Design review of the part shown in the three views and the two pictorial views. Dimensions are in mm from the part's minimum x, y and z. A direction names the side the tool comes from. Round coordinates to 2 decimals unless told otherwise and drop trailing zeros. Order: outer loops, then holes, each group sorted by start corner. A loop starts at its lowest first (then second) coordinate and runs counter-clockwise, first axis right, second up.
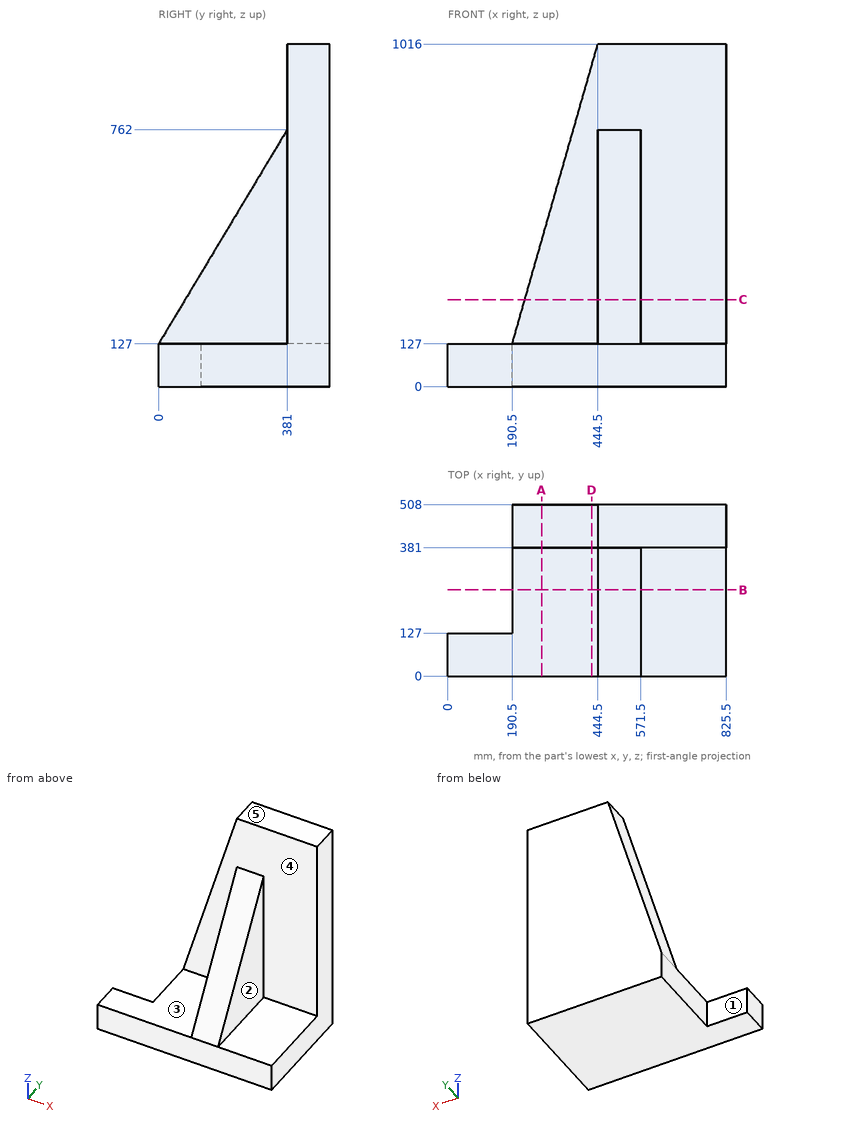
(1) Insertion check: pin 1 (6 mm diameter, centred on y = 352.5, z = 631.5, fed in from -X); pin 2 (8 mm diameter, centred on x = 455, y = 335.5, fed in from +Z); pin 3 (1.5 mm diameter, centred on y = 280, z = 367, fed in from +X). Each pin has a flat end and moves straight along its axis. Give the tip position at first contact, or say it passes through.
Data:
pin 1: stops at x = 444.5
pin 2: stops at z = 692.83
pin 3: stops at x = 571.5
(2) For the marked faces 1, 2, 3, 4 and 5, list the 3-axis set-ups (+Z, -Z, +X, -X, +Y, -Y) from which the entire face can be reached by the end or side of a thin tool; tool diameter is ignored.
Data:
face 1: +Z, -Z, -X, +Y
face 2: +Z, +X, -Y
face 3: +Z, -X, -Y
face 4: +Z, -Y
face 5: +Z, +X, -X, +Y, -Y
(3) Consider section A-A (x = 278). Write out the cut boundary in (y, z), and give its area (3 significant figures).
Data:
outline: (0, 0) - (508, 0) - (508, 433.25) - (381, 433.25) - (381, 127) - (0, 127) - close
area: 103,000 mm2
(4) Consider section D-D (x = 426). Write out the cut boundary in (y, z).
Data:
outline: (0, 0) - (508, 0) - (508, 951.25) - (381, 951.25) - (381, 127) - (0, 127) - close
(5) Consider section B-B (y = 255). Write out the cut boundary in (x, z).
Data:
outline: (190.5, 0) - (825.5, 0) - (825.5, 127) - (571.5, 127) - (571.5, 552) - (444.5, 552) - (444.5, 127) - (190.5, 127) - close
(6) To check wall thickness, follow probe 1 along Z at (x, y) = (657, 51.5); probe 2 along X at (y, z) = (274, 263); probe 3 along Y at (x, z) = (707, 299). State the ranges of each line that lie inside material, in increasing order.
Data:
probe 1: z = 0 to 127
probe 2: x = 444.5 to 571.5
probe 3: y = 381 to 508
(7) Consider section C-C (z = 258). Write out the cut boundary in (x, y).
Data:
outline: (227.93, 381) - (444.5, 381) - (444.5, 78.6) - (571.5, 78.6) - (571.5, 381) - (825.5, 381) - (825.5, 508) - (227.93, 508) - close
